Can you work these out from the drawing? Everything is in mm from the part's minimum corner. A direction names the side the tool comes from. Round coordinates to 2 decimals unless told otherwise and drop trailing zeros. Loops run counter-clockwise (first coordinate to the right, second up) from the corner with the lowest first, then second, coordinate; pieces in that order, holes last. Notation, with made-up numbers: M 58,53 L 93,53 A8 ccw 93,62 Z; hole C 77,33.25 d10. An arc over 180 degrees is marked long. Answer in a Markdown table with one row per item.
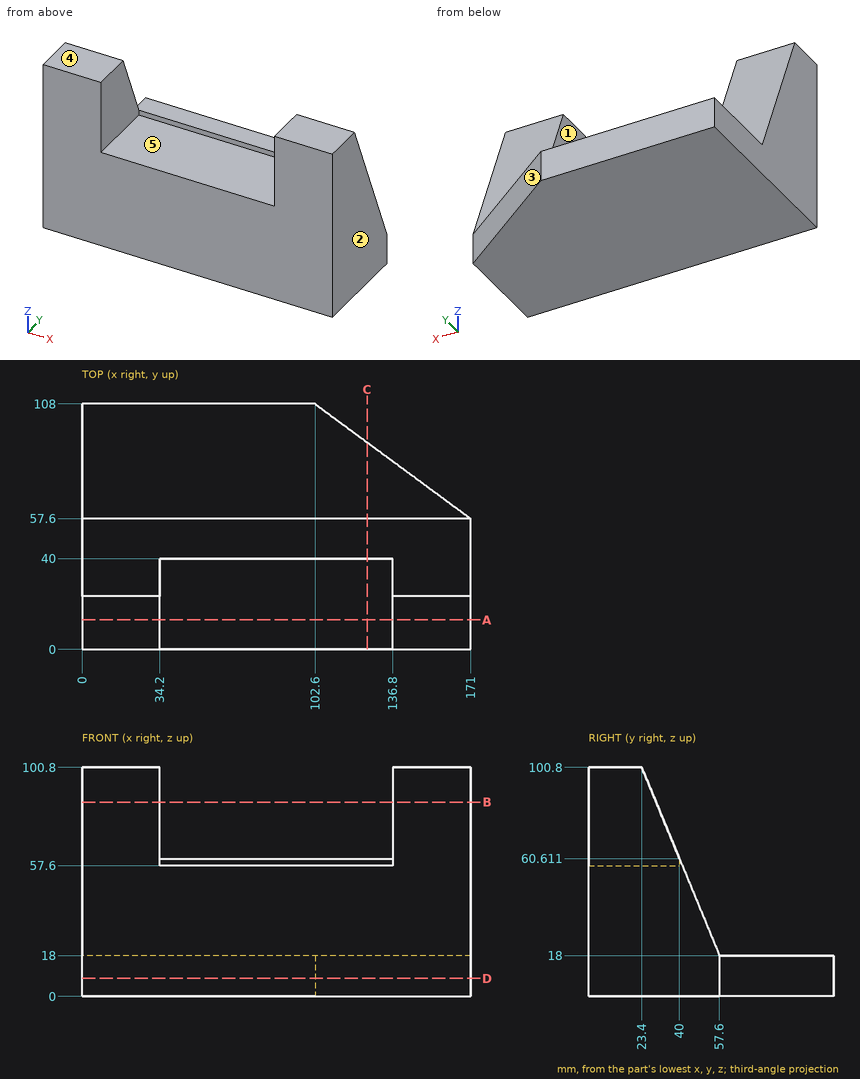
1) Which directions (+Z, -Z, +X, -X, +Y, -Y) give clear straight access to the entire face, cutting with the end or side of a thin tool? Please do the marked faces 1 and 2.
Computed:
| item | result |
|---|---|
| face 1 | +Z, -Y |
| face 2 | +Z, -Z, +X, +Y, -Y |
2) I want a section at B-B, the plane z = 85.5. Please give me the cut outline in (x, y).
Computed:
| item | result |
|---|---|
| outline | M 0,0 L 34.2,0 L 34.2,29.72 L 0,29.72 Z; M 136.8,0 L 171,0 L 171,29.72 L 136.8,29.72 Z |
3) If we mould it in two halves opening along X, with no side actions, what happens to the marked faces 3, 4 and 5? For each: released by +X, released by -X, zero draft, split by the parting line, or undercut.
Computed:
| item | result |
|---|---|
| face 3 | released by +X |
| face 4 | zero draft |
| face 5 | undercut |
4) I want a section at D-D, the plane z = 8. Please give me the cut outline in (x, y).
Computed:
| item | result |
|---|---|
| outline | M 0,0 L 171,0 L 171,57.6 L 102.6,108 L 0,108 Z |
5) I need wall thicknesses on line 1 (Z direction, x = 65, y = 10.5); line 2 (Y direction, x = 20, z = 60.5) (1 decimal); line 3 (Y direction, x = 13, z = 84.5). Which ranges of each line are inside material? Lowest first, please.
Computed:
| item | result |
|---|---|
| line 1 | z = 0 to 57.6 |
| line 2 | y = 0 to 40 |
| line 3 | y = 0 to 30.13 |
6) I want a section at C-C, the plane x = 125.5. Please give me the cut outline in (y, z).
Computed:
| item | result |
|---|---|
| outline | M 0,0 L 91.13,0 L 91.13,18 L 57.6,18 L 40,60.61 L 40,57.6 L 0,57.6 Z |
7) I want a section at A-A, the plane y = 13. Please give me the cut outline in (x, z), plus the area to 3 significant figures.
Computed:
| item | result |
|---|---|
| outline | M 0,0 L 171,0 L 171,100.8 L 136.8,100.8 L 136.8,57.6 L 34.2,57.6 L 34.2,100.8 L 0,100.8 Z |
| area | 12,800 mm² |
8) Will these pins go through, and if not, where does the flat tip stop? P1, Ø25, axis at x = 107.5, y = 88, coming from the +Z side; P2, Ø1.5, axis at x = 72, z = 58.5, coming from the -Y side; P3, Ø12, axis at y = 87.5, z = 17, coming from the -X side; P4, Ø6, axis at x = 106.5, z = 14.5, coming from the +Y side.
Computed:
| item | result |
|---|---|
| P1 | stops at z = 18 |
| P2 | stops at y = 40 |
| P3 | stops at x = 0 |
| P4 | stops at y = 107.34 |
